Part model, mm, in its own coordinate system. Face numbers are marked on the shaded views. Coordinates: 2 decimals unless noted, no trailing zeros. Loops run counter-clockwise (first coordinate to the right, second up) from the corner with the lowest first, then second, coordinate; pieces in that order, holes last.
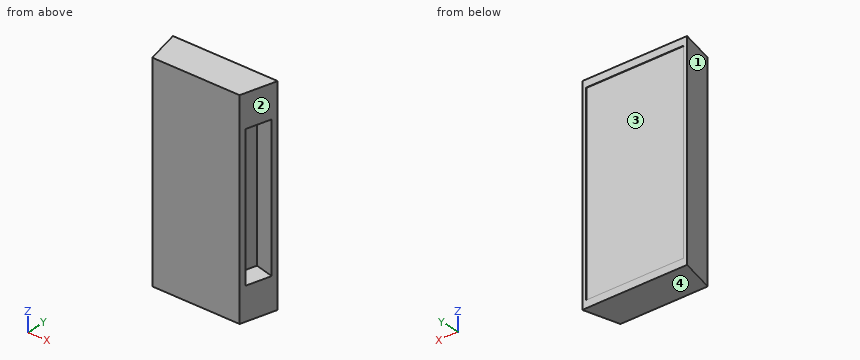
```python
from build123d import *

# Parameters (mm, degrees)
F1_DEPTH = 1750
F2_W     = 835.971278
F2_H     = 1625.499708
F3_DEPTH = 5
F4_W     = 211.788026
F4_H     = 1198.5433
F5_DEPTH = 165


with BuildPart() as f1:
    # F0 (on Top) → F1 (new body)
    with BuildSketch(Plane.XY):
        Polygon((-488.9687, 205.970883), (-413.9687, -94.029117), (336.0313, -94.029117), (411.0313, 205.970883), (-38.9687, 205.970883), align=None)
    extrude(amount=F1_DEPTH)

    # F2 (on face) → F3 (cut)
    with BuildSketch(Plane(origin=(0, 205.970883, 0), x_dir=(-1, 0, 0), z_dir=(0, 1, 0))):
        with Locations((38.9687, 875)):
            Rectangle(F2_W, F2_H)
    extrude(amount=-F3_DEPTH, mode=Mode.SUBTRACT)

    # F4 (on face) → F5 (cut)
    with BuildSketch(Plane(origin=(338.389251, -84.597313, 0), x_dir=(0.242536, 0.970143, 0), z_dir=(0.970143, -0.242536, 0))):
        with Locations((144.89438, 875)):
            Rectangle(F4_W, F4_H)
    extrude(amount=-F5_DEPTH, mode=Mode.SUBTRACT)


solid = f1.part
```
Q1. Drop flat-ended pins along their axis: P1, Ø1.5, axis at y = 29, z = 769, coming from the -X side; P2, Ø12, axis at y = 81, z = 421.5, coming from the -X side; P3, Ø4, axis at y = 145, z = 450.5, coming from the -X side. Give the stop position or say it passes through.
Q2. Saw through at C-C (y = 178). List the corners of the cut face in (x, z), plus the area to 3 significant figures.
Q3. Mould opens along X. For the marked faces 1, 2, 3 and 4 say: released by +X, released by -X, zero draft, split by the parting line, or undercut.
Q4. Probe line 1 (Y direction, x = 234.5, z = 181.5); line 2 (Y direction, x = 261.5, z = 435.5); line 3 (Y direction, x = 268, z = 1142.5). List the from-to ranges inside material, lowest first.
Q5. Saw through at A-A (z = 1378). List the corners of the cut face in (x, y).
Q6. Saw through at B-B (x = -36.5). List the corners of the cut face in (y, z), plus the area to 3 significant figures.
Q7. Saw through at D-D (y = 106). List the corners of the cut face in (x, z), plus the area to 3 significant figures.
Checked values:
1. P1: stops at x = -444.91
1. P2: stops at x = -459.23
1. P3: stops at x = -474.23
2. outline: (-481.98, 0) - (404.04, 0) - (404.04, 1750) - (-481.98, 1750) - close; hole (233.96, 275.73) - (322.03, 275.73) - (322.03, 1474.27) - (233.96, 1474.27) - close
2. area: 1,440,000 mm2
3. face 1: released by -X
3. face 2: released by +X
3. face 3: undercut
3. face 4: zero draft
4. line 1: y = -94.03 to 200.97
4. line 2: y = -94.03 to -25.17, 193.13 to 200.97
4. line 3: y = -94.03 to -26.8, 191.51 to 200.97
5. outline: (-488.97, 205.97) - (-413.97, -94.03) - (336.03, -94.03) - (347.85, -46.76) - (187.77, -6.74) - (239.14, 198.72) - (399.21, 158.7) - (411.03, 205.97) - (379.02, 205.97) - (379.02, 200.97) - (-456.95, 200.97) - (-456.95, 205.97) - close
6. outline: (-94.03, 0) - (205.97, 0) - (205.97, 62.25) - (200.97, 62.25) - (200.97, 1687.75) - (205.97, 1687.75) - (205.97, 1750) - (-94.03, 1750) - close
6. area: 517,000 mm2
7. outline: (-463.98, 0) - (386.04, 0) - (386.04, 275.73) - (215.96, 275.73) - (215.96, 1474.27) - (386.04, 1474.27) - (386.04, 1750) - (-463.98, 1750) - close
7. area: 1,280,000 mm2
